Job drawing, mm, ordinate dimensions from the low corner. One solid piece. Give positions to 0.01 mm unless a question says otherwise; leave off trailing zeros. Write each loop counter-clockwise with the first axis right and the second up, starting at its lowest first coordinate (ties: lowest second). Pieces come first, ordered by that corner, then holes. Notation, with made-up numbers: (2, 65.5) -> (48, 65.5) arc R13 ccw to (48, 69.5) -> close; hole circle Ø6 at (-39.75, -25). An arc over 180 degrees is marked (long way). Put each result on its own line as item: value. Start each with the question number.
Item 1: Slice it at A-A, the plane y = 2.25. List the corners of the cut face in (x, z), plus the area to 3 significant figures.
Item 2: Slice it at B-B, the plane x = 5. List the corners of the cut face in (y, z), plus the area to 3 significant figures.
Item 3: Slice it at C-C, the plane z = 5. List the corners of the cut face in (x, y).
Item 4: Drill centre lines: line 1 along X through (y, z) = (1.5, 75); line 2 along Z through (x, y) = (115, 2.45); line 3 along X through (y, z) = (1.25, 72.5). Where is each one in solid material? Low to high.
Item 5: Flat gauge pin, fed straight in: pin 1 Ø4 at (x, z) = (6.5, 6) entering from +Y. Where does the tip first touch, or does it go through?
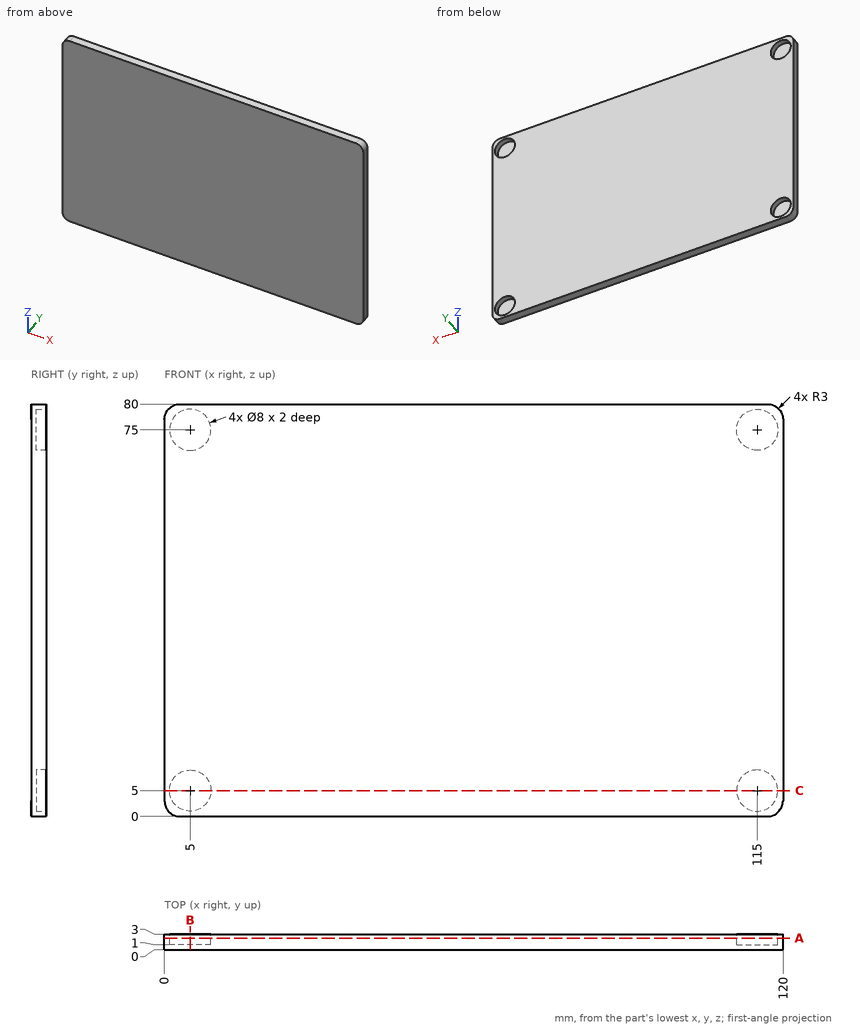
Values follow:
1. outline: (0, 3) arc R3 ccw to (3, 0) -> (117, 0) arc R3 ccw to (120, 3) -> (120, 77) arc R3 ccw to (117, 80) -> (3, 80) arc R3 ccw to (0, 77) -> close; hole circle Ø8 at (5, 5); hole circle Ø8 at (5, 75); hole circle Ø8 at (115, 5); hole circle Ø8 at (115, 75)
1. area: 9,390 mm2
2. outline: (0, 0) -> (3, 0) -> (3, 1) -> (1, 1) -> (1, 9) -> (3, 9) -> (3, 71) -> (1, 71) -> (1, 79) -> (3, 79) -> (3, 80) -> (0, 80) -> close
2. area: 208 mm2
3. outline: (0, 0) -> (120, 0) -> (120, 3) -> (119, 3) -> (119, 1) -> (111, 1) -> (111, 3) -> (9, 3) -> (9, 1) -> (1, 1) -> (1, 3) -> (0, 3) -> close
4. line 1: 0 to 1, 9 to 111, 119 to 120
4. line 2: 0 to 1, 9 to 71, 79 to 80
4. line 3: 0 to 1.88, 8.12 to 111.88, 118.12 to 120
5. pin 1: y = 1
